Model file for the job. Use its own axes, mm. Round coordinates to 2 decimals unless told otherwise and drop trailing zeros. Loops run counter-clockwise (first coordinate to the right, second up) from the corner with the lowest first, then second, coordinate; pieces in that order, holes last. Notation, with made-up numbers: (78.25, 12) -> (134.25, 12) arc R19 cw to (134.25, 45) -> close; hole circle Ø4 at (10.5, 13.25). An arc over 180 degrees is marked (long way). Use a Markdown table: item, result. Add a question column.
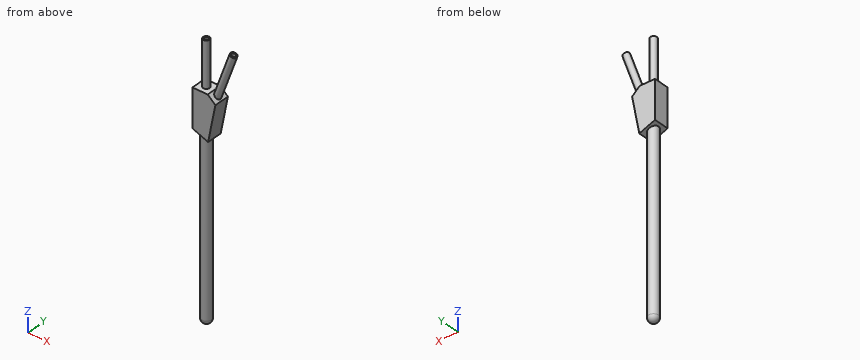
```python
from build123d import *
from build123d.topology import SkipClean

# Parameters (mm, degrees)
BOSS_EXTRUDE1_DEPTH = 6
SKETCH4_R           = 2
BOSS_EXTRUDE2_DEPTH = 71.5
FILLET1_R           = 2
SKETCH5_R           = 1.25
BOSS_EXTRUDE3_DEPTH = 17.7
SKETCH7_R           = 1.25
BOSS_EXTRUDE4_DEPTH = 18.5
BOSS_EXTRUDE5_START = -5
SKETCH7_2_R         = 1.25
BOSS_EXTRUDE5_DEPTH = 5
SHELL1_START        = 0.5
SHELL1_DEPTH        = 5
SHELL1_START_2      = 14.5
SHELL1_2_OUTLINE_R  = 0.75
SHELL1_2_DEPTH      = 18.2
SHELL1_START_3      = 14.294760558
SHELL1_3_OUTLINE_R  = 0.75
SHELL1_3_DEPTH      = 19.602760214


with BuildPart() as part:
    # Sketch1 → Boss-Extrude1 (new body)
    with BuildSketch(Plane(origin=(0, 0, 0), x_dir=(1, 0, 0), z_dir=(0, 1, 0))):
        Polygon((0, 0), (6.158217776, 2.374100634), (9, -12.354248689), (6, -15), (0, -15), align=None)
    extrude(amount=BOSS_EXTRUDE1_DEPTH)

    # Sketch4 → Boss-Extrude2 (add)
    with BuildSketch(Plane.XY):
        with Locations((3.079108888, 3)):
            Circle(SKETCH4_R)
    extrude(amount=-BOSS_EXTRUDE2_DEPTH)

    # Fillet1
    fillet1_edges = [part.edges().sort_by_distance(p)[0] for p in [
        (1.079108888, 3, -71.5),
    ]]
    fillet(fillet1_edges, radius=FILLET1_R)

    # Sketch5 → Boss-Extrude3 (add)
    with BuildSketch(Plane.XY.offset(15)):
        with Locations((3, 3)):
            Circle(SKETCH5_R)
    extrude(amount=BOSS_EXTRUDE3_DEPTH)

    # Sketch7 → Boss-Extrude4 (add)
    with BuildSketch(Plane(origin=(7.5, 6, 13.677124344), x_dir=(0.9424618522341062, 0, -0.33431371058252735), z_dir=(0.33431371058252735, 0, 0.9424618522341062))):
        with Locations(Location((0.000948247, -3, 0), (0, 0, 90.043464463))):
            Circle(SKETCH7_R)
    extrude(amount=BOSS_EXTRUDE4_DEPTH)

    # Sketch7_2 → Boss-Extrude5 (add)
    with SkipClean():  # the faces are left unmerged after this step: merging them gives an invalid solid
        with BuildSketch(Plane(origin=(7.5, 6, 13.677124344), x_dir=(0.9424618522341062, 0, -0.33431371058252735), z_dir=(0.33431371058252735, 0, 0.9424618522341062)).offset(BOSS_EXTRUDE5_START)):
            with Locations((0.000948247, -3)):
                Circle(SKETCH7_2_R)
        extrude(amount=BOSS_EXTRUDE5_DEPTH)

    # Shell1: read off the stored shape, not the designer's step
    # Shell1 outline → Shell1 (cut)
    with SkipClean():  # the faces are left unmerged after this step: merging them gives an invalid solid
        with BuildSketch(Plane(origin=(0, 0, 0), x_dir=(1, 0, 0), z_dir=(0, 1, 0)).offset(SHELL1_START)):
            Polygon((5.811017763, -14.5), (8.454902336, -12.168312975), (5.780487015, 1.692609497), (0.5, -0.343110582), (0.5, -14.5), align=None)
        extrude(amount=SHELL1_DEPTH, mode=Mode.SUBTRACT)

    # Shell1 2 outline → Shell1 2 (cut)
    with SkipClean():  # the faces are left unmerged after this step: merging them gives an invalid solid
        with BuildSketch(Plane.XY.offset(SHELL1_START_2)):
            with Locations((3, 3)):
                Circle(SHELL1_2_OUTLINE_R)
        extrude(amount=SHELL1_2_DEPTH, mode=Mode.SUBTRACT)

    # Shell1 3 outline → Shell1 3 (cut)
    with SkipClean():  # the faces are left unmerged after this step: merging them gives an invalid solid
        with BuildSketch(Plane(origin=(0, 0, 0), x_dir=(0.9424618522341063, 0, -0.3343137105825272), z_dir=(0.3343137105825271, 0, 0.9424618522341063)).offset(SHELL1_START_3)):
            with Locations((2.496961949, 3)):
                Circle(SHELL1_3_OUTLINE_R)
        extrude(amount=SHELL1_3_DEPTH, mode=Mode.SUBTRACT)

    # Shell1 4 outline → Shell1 4 (revolve, cut)
    with SkipClean():  # the faces are left unmerged after this step: merging them gives an invalid solid
        with BuildSketch(Plane(origin=(3.079108888, 3, 0), x_dir=(1, 0, 0), z_dir=(0, -1, 0))):
            with BuildLine():
                ThreePointArc((0, -71), (1.060660172, -70.560660171), (1.5, -69.499999999))
                Line((1.5, -69.499999999), (1.5, -0.072605564))
                Line((1.5, -0.072605564), (0, -0.072605564))
                Line((0, -0.072605564), (0, -71))
            make_face()
        revolve(axis=Axis((3.079108888, 3, 0), (0, 0, 1)), mode=Mode.SUBTRACT)


solid = part.part
```
1) Cut at C-C on z = 16. Count the separate pieces of the cut face and the enclosed holes in it, and give its area (4 significant figures).
2) Pin check, flat tips, straight feed: pin 1 Ø3 at (x, y) = (7, 4) entering from -Z; pin 2 Ø1.5 at (y, z) = (5, 11.5) entering from +X; pin 3 Ø1 at (y, z) = (5, -4) entering from +X; pin 4 Ø3 at (x, z) = (7, -51.5) entering from -Y. Stop position of each tip, or through.
3) Wall check: probe 1 along Y at (x, z) = (3, 18.5); probe 2 along X at (y, z) = (2.9, -5); probe 3 along X at (y, z) = (2.9, 21). Give the ranges that are in metal, low to high. Write a range as from..to.
4) Cut at B-B on z = -21. Write the cut outline in (x, y), and give its area (3 significant figures).
5) Cut at A-A on z = 2. Write the cut outline in (x, y), and give its area (3 significant figures).
Established:
| question | item | result |
|---|---|---|
| 1 | separate pieces | 2 |
| 1 | enclosed holes | 2 |
| 1 | area | 6.475 mm^2 |
| 2 | pin 1 | stops at z = -2.37 |
| 2 | pin 2 | stops at x = 8.98 |
| 2 | pin 3 | stops at x = 4.4 |
| 2 | pin 4 | passes through |
| 3 | probe 1 | y = 1.75..2.25, 3.75..4.25 |
| 3 | probe 2 | x = 1.08..1.58, 4.58..5.08 |
| 3 | probe 3 | x = 1.75..2.26, 3.74..4.25, 8.78..9.31, 10.89..11.42 |
| 4 | outline | circle Ø4 at (3.08, 3); hole circle Ø3 at (3.08, 3) |
| 4 | area | 5.50 mm^2 |
| 5 | outline | (0, 0) -> (7, 0) -> (7, 6) -> (0, 6) -> close; hole (0.5, 0.5) -> (6.49, 0.5) -> (6.49, 5.5) -> (0.5, 5.5) -> close |
| 5 | area | 12.0 mm^2 |
